Source: CAD feature listing. Evaluate the final solid. Frame: model axes, mm. A direction names the side the tool comes from. Coordinates: 2 decimals unless noted, no trailing zeros. Loops run counter-clockwise (first coordinate to the right, second up) from the corner with the lowest first, then second, coordinate; pieces in that order, holes last. Notation, with made-up numbers: (-5, -17) - (31, -17) arc R13 cw to (31, 6) - close; hole circle Ø10 at (9.5, 39). An arc over 180 degrees is marked (long way). Use one line per item in the form item = value. Start each with the question number.
from build123d import *

# Parameters (mm, degrees)
SKETCH1_R           = 2.975
BOSS_EXTRUDE1_DEPTH = 50
SKETCH2_W           = 10.000004986
SKETCH2_H           = 10.000004986
BOSS_EXTRUDE2_DEPTH = 10
FILLET1_R           = 1
CHAMFER1_SIZE       = 0.5


with BuildPart() as part:
    # Sketch1 → Boss-Extrude1 (new body)
    with BuildSketch(Plane(origin=(0, 0, 0), x_dir=(1, 0, 0), z_dir=(0, 1, 0))):
        with Locations(Location((0, 0, 0), (0, 0, 270))):
            Circle(SKETCH1_R)
    extrude(amount=BOSS_EXTRUDE1_DEPTH)

    # Sketch2 → Boss-Extrude2 (add, symmetric)
    with BuildSketch(Plane.XY):
        Rectangle(SKETCH2_W, SKETCH2_H)
    extrude(amount=BOSS_EXTRUDE2_DEPTH, both=True)

    # Fillet1
    fillet1_edges = [part.edges().sort_by_distance(p)[0] for p in [
        (0, 50, -2.975),
        (0, 5.000002493, -2.975),
        (5.000002493, 0, -10),
        (0, 5.000002493, -10),
        (5.000002493, 5.000002493, 0),
        (-5.000002493, 0, -10),
        (-5.000002493, 5.000002493, 0),
        (5.000002493, 0, 10),
        (0, 5.000002493, 10),
        (-5.000002493, 0, 10),
    ]]
    fillet(fillet1_edges, radius=FILLET1_R)

    # Chamfer1
    chamfer1_edges = [part.edges().sort_by_distance(p)[0] for p in [
        (0, -5.000002493, 10),
        (0, -5.000002493, -10),
        (5.000002493, -5.000002493, 0),
        (-5.000002493, -5.000002493, 0),
        (4.707109274, -5.000002493, 9.707106781),
        (4.707109274, -5.000002493, -9.707106781),
        (-4.707109274, -5.000002493, -9.707106781),
        (-4.707109274, -5.000002493, 9.707106781),
    ]]
    chamfer(chamfer1_edges, length=CHAMFER1_SIZE)


solid = part.part
(1) Access query for faces 1 (the face through (4.49, -4.8, 9.5)), 2 (the face through (0.89, 27.2, 2.84)). Directions: +Z, -Z, +X, -X, +Y, -Y. A direction counts if a zero-diameter tool reaches every point of the face in a straight line with its end or side. Return the directions, or none.
(2) Cut plane D-D, the plane y = 21.5. Output: boundary loops of the cut face in (x, z) (3 decimals).
(3) Cut plane B-B, the plane z = -5. Output: boundary loops of the cut face in (x, y).
(4) Cut plane A-A, the plane x = 0. Output: boundary loops of the cut face in (y, z) (3 decimals), plus the area to 3 significant figures.
(5) Cut plane C-C, the plane z = 0. Output: boundary loops of the cut face in (x, y) (3 decimals), plus the area to 3 significant figures.
(6) Material intervals for line 1 (Y direction, x = -3.5, z = -7.75); line 2 (X direction, y = 6.5, z = 0) (3 decimals); line 3 (Z direction, x = 1.75, y = 17), sorted ascending.
(7) Contact query for flat-ended pins moving along their axis: pin 1 (12 mm diameter, centred on y = 40, z = 0, fed in from -X) (3 decimals); pin 2 (4 mm diameter, centred on y = 38.5, z = 6.5, fed in from +X); pin 3 (1.5 mm diameter, centred on x = -1.5, z = 6.5, fed in from +Y); pin 4 (3 mm diameter, centred on x = 1, y = 11, fed in from -Z) (3 decimals). Output: stop coordinate, or through.
Recorded:
q1.face_1 = +Z, +X, -Y
q1.face_2 = +Y
q2.outline = circle Ø5.95 at (0, 0)
q3.outline = (-5, -4.5) - (-4.5, -5) - (4.5, -5) - (5, -4.5) - (5, 4) arc R1 ccw to (4, 5) - (-4, 5) arc R1 ccw to (-5, 4) - close
q4.outline = (-5, -9.5) - (-4.5, -10) - (4, -10) arc R1 ccw to (5, -9) - (5, -3.975) arc R1 cw to (6, -2.975) - (49, -2.975) arc R1 ccw to (50, -1.975) - (50, 1.975) arc R1 ccw to (49, 2.975) - (6, 2.975) arc R1 cw to (5, 3.975) - (5, 9) arc R1 ccw to (4, 10) - (-4.5, 10) - (-5, 9.5) - close
q4.area = 467 mm²
q5.outline = (-5, -4.5) - (-4.5, -5) - (4.5, -5) - (5, -4.5) - (5, 4) arc R1 ccw to (4, 5) - (3.975, 5) arc R1 cw to (2.975, 6) - (2.975, 49) arc R1 ccw to (1.975, 50) - (-1.975, 50) arc R1 ccw to (-2.975, 49) - (-2.975, 6) arc R1 cw to (-3.975, 5) - (-4, 5) arc R1 ccw to (-5, 4) - close
q5.area = 367 mm²
q6.line_1 = -5 to 5
q6.line_2 = -2.975 to 2.975
q6.line_3 = -2.41 to 2.41
q7.pin_1 = -2.975
q7.pin_2 = through
q7.pin_3 = 5
q7.pin_4 = -2.975
